The listing builds one solid part. Answer for the finished solid, in the listing's coordinates (mm). A direction names the side the tool comes from. Coordinates: 2 decimals unless noted, no trailing zeros. Write each loop counter-clockwise with the first axis right and the second up, starting at its lowest first coordinate (ties: lowest second). Pieces come first, ordered by that corner, then holes. Notation, with made-up numbers: M 49.5,28 L 103.5,28 A9 ccw 103.5,40 Z; hole C -9,76 d4. An arc over 180 degrees is marked long. Answer as CSV lines item,"result".
```python
from build123d import *

# Parameters (mm, degrees)
SKETCH1_W           = 54.102
SKETCH1_H           = 55.88
BOSS_EXTRUDE1_DEPTH = 2.54
SKETCH2_R           = 0.762
CUT_EXTRUDE1_DEPTH  = 49.276


with BuildPart() as part:
    # Sketch1 → Boss-Extrude1 (new body)
    with BuildSketch(Plane(origin=(0, 0, 0), x_dir=(1, 0, 0), z_dir=(0, 1, 0))):
        with Locations((27.051, 27.94)):
            Rectangle(SKETCH1_W, SKETCH1_H)
    extrude(amount=BOSS_EXTRUDE1_DEPTH)

    # Sketch2 → Cut-Extrude1 (cut)
    with BuildSketch(Plane(origin=(0, 2.54, 0), x_dir=(1, 0, 0), z_dir=(0, 1, 0))):
        with Locations(Location((1.27, 54.61, 0), (0, 0, 270))):
            Circle(SKETCH2_R)
        with Locations(Location((52.832, 1.27, 0), (0, 0, 270))):
            Circle(SKETCH2_R)
        with BuildLine():
            Line((6.096, 49.53), (6.096, 6.35))
            ThreePointArc((6.096, 6.35), (4.572, 4.826), (3.048, 6.35))
            Line((3.048, 6.35), (3.048, 49.53))
            ThreePointArc((3.048, 49.53), (4.572, 51.054), (6.096, 49.53))
        make_face()
        with BuildLine():
            Line((11.176, 49.53), (11.176, 6.35))
            ThreePointArc((11.176, 6.35), (9.652, 4.826), (8.128, 6.35))
            Line((8.128, 6.35), (8.128, 49.53))
            ThreePointArc((8.128, 49.53), (9.652, 51.054), (11.176, 49.53))
        make_face()
        with BuildLine():
            Line((16.256, 49.53), (16.256, 6.35))
            ThreePointArc((16.256, 6.35), (14.732, 4.826), (13.208, 6.35))
            Line((13.208, 6.35), (13.208, 49.53))
            ThreePointArc((13.208, 49.53), (14.732, 51.054), (16.256, 49.53))
        make_face()
        with BuildLine():
            Line((21.336, 49.53), (21.336, 6.35))
            ThreePointArc((21.336, 6.35), (19.812, 4.826), (18.288, 6.35))
            Line((18.288, 6.35), (18.288, 49.53))
            ThreePointArc((18.288, 49.53), (19.812, 51.054), (21.336, 49.53))
        make_face()
        with BuildLine():
            Line((26.416, 49.53), (26.416, 6.35))
            ThreePointArc((26.416, 6.35), (24.892, 4.826), (23.368, 6.35))
            Line((23.368, 6.35), (23.368, 49.53))
            ThreePointArc((23.368, 49.53), (24.892, 51.054), (26.416, 49.53))
        make_face()
        with BuildLine():
            Line((31.496, 49.53), (31.496, 6.35))
            ThreePointArc((31.496, 6.35), (29.972, 4.826), (28.448, 6.35))
            Line((28.448, 6.35), (28.448, 49.53))
            ThreePointArc((28.448, 49.53), (29.972, 51.054), (31.496, 49.53))
        make_face()
        with BuildLine():
            Line((36.576, 49.53), (36.576, 6.35))
            ThreePointArc((36.576, 6.35), (35.052, 4.826), (33.528, 6.35))
            Line((33.528, 6.35), (33.528, 49.53))
            ThreePointArc((33.528, 49.53), (35.052, 51.054), (36.576, 49.53))
        make_face()
        with BuildLine():
            Line((41.656, 49.53), (41.656, 6.35))
            ThreePointArc((41.656, 6.35), (40.132, 4.826), (38.608, 6.35))
            Line((38.608, 6.35), (38.608, 49.53))
            ThreePointArc((38.608, 49.53), (40.132, 51.054), (41.656, 49.53))
        make_face()
        with BuildLine():
            Line((46.736, 49.53), (46.736, 6.35))
            ThreePointArc((46.736, 6.35), (45.212, 4.826), (43.688, 6.35))
            Line((43.688, 6.35), (43.688, 49.53))
            ThreePointArc((43.688, 49.53), (45.212, 51.054), (46.736, 49.53))
        make_face()
        with BuildLine():
            Line((51.816, 49.53), (51.816, 6.35))
            ThreePointArc((51.816, 6.35), (50.292, 4.826), (48.768, 6.35))
            Line((48.768, 6.35), (48.768, 49.53))
            ThreePointArc((48.768, 49.53), (50.292, 51.054), (51.816, 49.53))
        make_face()
    extrude(amount=-CUT_EXTRUDE1_DEPTH, mode=Mode.SUBTRACT)


solid = part.part
```
Q1. Straight lines are drawn through the part: line 1 (X direction, y = 1.25, z = -1.27); line 2 (X direction, y = 1.4, z = -54.61); line 3 (Z direction, x = 50.5, y = 1.9). For each, find the intervals that lie inside material, in ascending order.
Output:
line 1,"0 to 52.07, 53.59 to 54.1"
line 2,"0 to 0.51, 2.03 to 54.1"
line 3,"-55.88 to -51.04, -4.84 to 0"
Q2. For faces 1 (the flat face through (0, 1, -28)), 2 (the cylindrical face through (40.166, 1.288, -4.826)), determine the directions among +Z, -Z, +X, -X, +Y, -Y from which every point of the face is accessible in a straight line to the end or side of a thin tool.
Output:
face 1,"+Z, -Z, -X, +Y, -Y"
face 2,"+Y, -Y"
Q3. The mould has two halves that part along Z. Classify faces 3 (the flat face through (27, 0, -28)), 4 (the flat face through (8.128, 1, -28)): pulls with the +Z half, pulls with the -Z half, needs draft (parallel to the pull), parting line crosses it, or undercut.
Output:
face 3,"needs draft"
face 4,"undercut"
Q4. Find section B-B (x = 1.27). Give the vertices of the cut face in (y, z).
Output:
outline,"M 0,-55.88 L 2.54,-55.88 L 2.54,-55.37 L 0,-55.37 Z; M 0,-53.85 L 2.54,-53.85 L 2.54,0 L 0,0 Z"
Q5. Find section C-C (z = -7.5). Count the separate pieces of the cut face and the enclosed holes in it, and give its area (3 significant figures).
Output:
separate pieces,"11"
enclosed holes,"0"
area,"60.0 mm2"
Q6. Find section A-A (z = -54.61). Give the vertices of the cut face in (x, y).
Output:
outline,"M 0,0 L 0.51,0 L 0.51,2.54 L 0,2.54 Z; M 2.03,0 L 54.1,0 L 54.1,2.54 L 2.03,2.54 Z"
